```python
from build123d import *

# Parameters (mm, degrees)
SKETCH1_R           = 36.871673704
BOSS_EXTRUDE1_DEPTH = 26.416
SKETCH2_R           = 4.719401224
SKETCH2_R_2         = 3.956193561
SKETCH2_R_3         = 6.025487418
CUT_EXTRUDE1_DEPTH  = 5.08
CHAMFER1_SIZE       = 1
SKETCH4_W           = 30
SKETCH4_H           = 20
CUT_EXTRUDE2_DEPTH  = 10
FILLET1_R           = 4
FILLET3_R           = 2
CHAMFER3_SIZE       = 1


with BuildPart() as part:
    # Sketch1 → Boss-Extrude1 (new body)
    with BuildSketch(Plane(origin=(0, 0, 0), x_dir=(1, 0, 0), z_dir=(0, 1, 0))):
        with Locations(Location((0, 0, 0), (0, 0, 270))):  # turned: the seam where the file's is
            Circle(SKETCH1_R)
    extrude(amount=BOSS_EXTRUDE1_DEPTH)

    # Sketch2 → Cut-Extrude1 (cut)
    with BuildSketch(Plane(origin=(0, 26.416, 0), x_dir=(1, 0, 0), z_dir=(0, 1, 0))):
        with Locations(Location((-19.22121176, 13.655520005, 0), (0, 0, 270))):  # turned: the seam where the file's is
            Circle(SKETCH2_R)
        with Locations(Location((7.876648873, 14.748238638, 0), (0, 0, 270))):  # turned: the seam where the file's is
            Circle(SKETCH2_R_2)
        with Locations(Location((-1.786448021, -11.295248686, 0), (0, 0, 270))):  # turned: the seam where the file's is
            Circle(SKETCH2_R_3)
    extrude(amount=-CUT_EXTRUDE1_DEPTH, mode=Mode.SUBTRACT)

    # Chamfer1
    chamfer1_edges = [part.edges().sort_by_distance(p)[0] for p in [
        (0, 26.416, -36.871673704),
    ]]
    chamfer(chamfer1_edges, length=CHAMFER1_SIZE)

    # Sketch4 → Cut-Extrude2 (cut)
    with BuildSketch(Plane(origin=(0, 26.416, 0), x_dir=(1, 0, 0), z_dir=(0, 1, 0))):
        with Locations((30, 0)):
            Rectangle(SKETCH4_W, SKETCH4_H)
    extrude(amount=-CUT_EXTRUDE2_DEPTH, mode=Mode.SUBTRACT)

    # Fillet1
    fillet1_edges = [part.edges().sort_by_distance(p)[0] for p in [
        (15, 21.416, -10),
        (15, 21.416, 10),
    ]]
    fillet(fillet1_edges, radius=FILLET1_R)

    # Fillet3
    fillet3_edges = [part.edges().sort_by_distance(p)[0] for p in [
        (-1.786448021, 21.336, 5.269761268),
        (-19.22121176, 21.336, -18.374921228),
        (7.876648873, 21.336, -18.7044322),
    ]]
    fillet(fillet3_edges, radius=FILLET3_R)

    # Chamfer3
    chamfer3_edges = [part.edges().sort_by_distance(p)[0] for p in [
        (-1.786448021, 26.416, 5.269761268),
        (-19.22121176, 26.416, -18.374921228),
        (7.876648873, 26.416, -18.7044322),
    ]]
    chamfer(chamfer3_edges, length=CHAMFER3_SIZE)


solid = part.part
```
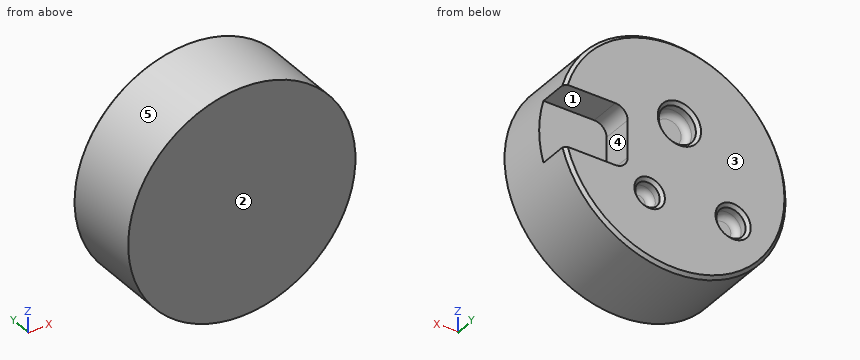
Geometry: final body of the model. Coordinates: model frame, mm. Face numbers are marked on the shaded views. A direction names the side the tool comes from. Coordinates: 2 decimals unless noted, no trailing zeros. Order: outer loops, then holes, each group sorted by start corner. A loop starts at its lowest first (then second) coordinate and runs counter-clockwise, first axis right, second up. Notation, with made-up numbers: (15.5, -27.75) - (44.5, -27.75) arc R16 ccw to (44.5, -8.75) - close; hole circle Ø6 at (11, -4). An arc over 180 degrees is marked (long way). Write each question's results on one line, items separated by ' | '.
1) Section B-B, the plane y = 8.5. Return loops of the section in (x, z), plus the area to 3 significant figures.
Results list:
outline: circle Ø73.74 at (0, 0) | area: 4,270 mm^2
2) Section A-A, the plane z = 0. Return loops of the section in (x, y), plus the area to 3 significant figures.
Results list:
outline: (-36.87, 0) - (36.87, 0) - (36.87, 16.42) - (15, 16.42) - (15, 26.42) - (-35.87, 26.42) - (-36.87, 25.42) - close | area: 1,730 mm^2
3) Pin query (flat end, axial travel): pin 1 (1.2 mm diameter, centred on x = 7.5, z = -14, fed in from +Y); pin 2 (6 mm diameter, centred on x = 25.5, z = 0, fed in from +Y); pin 3 (11 mm diameter, centred on y = 24, z = -0.5, fed in from +X). Return the tip coordinate at first contact, or that it passes through.
Results list:
pin 1: y = 21.34 | pin 2: y = 16.42 | pin 3: x = 15
4) Line query: line 1 (X direction, y = 24.75, z = -16); line 2 (Y direction, x = 17, z = 3); line 3 (Z direction, x = 22, y = 25). Output: solid intervals per line, ascending. Write a range as from..to.
Results list:
line 1: -33.22..-23.32, -15.13..4.12, 11.63..33.22 | line 2: 0..16.42 | line 3: -29.59..-10, 10..29.59
5) Pull-direction query (X, two-part tool) for the marked faces 3, 4 and 5; classes: pulls with the +X half, pulls with the -X half, needs draft (parallel to the pull), parting line crosses it, or undercut.
Results list:
face 3: needs draft | face 4: pulls with the +X half | face 5: parting line crosses it
6) Set-up query: the marked faces 1 and 2. Return all of +Z, -Z, +X, -X, +Y, -Y with unobstructed straight access to the full face (end or side cutting, diameter ignored); none if empty.
Results list:
face 1: +X, +Y | face 2: +Z, -Z, +X, -X, -Y
